Here's how the part is built. I have some questions about the finished solid (model axes, mm). A direction names the side the tool comes from. Round coordinates to 2 decimals unless told otherwise and drop trailing zeros. Order: outer loops, then holes, each group sorted by start corner. A loop starts at its lowest first (then second) coordinate and runs counter-clockwise, first axis right, second up. Notation, with made-up numbers: (35.25, 11) - (81.25, 11) arc R12 cw to (81.25, 21) - close; hole circle Ø9 at (77.25, 29.5). An arc over 180 degrees is marked (long way). Answer as a JSON object with one key per item and string values.
```python
from build123d import *
from build123d.topology import SkipClean

# Parameters (mm, degrees)
CROQUIS1_R              = 1.717841821
CROQUIS1_R_2            = 1.259750669
CROQUIS1_W              = 27.485469141
CROQUIS1_H              = 14.887962451
SALIENTE_EXTRUIR1_DEPTH = 5
SALIENTE_EXTRUIR2_START = -5
SALIENTE_EXTRUIR2_DEPTH = 5
CORTAR_EXTRUIR1_DEPTH   = 5
CORTAR_EXTRUIR2_DEPTH   = 2
CUT_EXTRUDE2_DEPTH      = 83.704538261


with BuildPart() as part:
    # Croquis1 → Saliente-Extruir1 (new body)
    with BuildSketch(Plane(origin=(0, 0, -2.5), x_dir=(-1, 0, 0), z_dir=(0, 0, -1))):
        with BuildLine():
            Line((2.183126414, 10.199004786), (2.457799007, 10.747834714))
            ThreePointArc((2.457799007, 10.747834714), (3.150356623, 11.03498533), (3.533498829, 10.390552574))
            Line((3.533498829, 10.390552574), (3.410556906, 9.704532228))
            Line((3.410556906, 9.704532228), (36.957948904, -3.17310503))
            ThreePointArc((36.957948904, -3.17310503), (40.309989238, -4.118478177), (43.778179918, -4.437160132))
            Line((43.778179918, -4.437160132), (75.884737747, -4.437160132))
            ThreePointArc((75.884737747, -4.437160132), (79.123931349, -3.095442211), (80.46564927, 0.143751392))
            Line((80.46564927, 0.143751392), (80.46564927, 13.886485962))
            ThreePointArc((80.46564927, 13.886485962), (79.123931349, 17.125679564), (75.884737747, 18.467397485))
            Line((75.884737747, 18.467397485), (43.778179918, 18.467397485))
            ThreePointArc((43.778179918, 18.467397485), (38.923372817, 17.631925595), (34.62713443, 15.221634951))
            ThreePointArc((34.62713443, 15.221634951), (27.84817952, 12.197288027), (20.46564927, 12.971336544))
            Line((20.46564927, 12.971336544), (6.293279019, 18.411599775))
            Line((6.293279019, 18.411599775), (6.008822105, 17.843219559))
            ThreePointArc((6.008822105, 17.843219559), (5.316264489, 17.556068943), (4.933122282, 18.200501699))
            Line((4.933122282, 18.200501699), (5.041383533, 18.804603367))
            ThreePointArc((5.041383533, 18.804603367), (4.263160644, 18.876341405), (3.484068945, 18.814751339))
            Line((3.484068945, 18.814751339), (3.584448287, 18.209290101))
            ThreePointArc((3.584448287, 18.209290101), (3.192940304, 17.56990522), (2.504183677, 17.866056933))
            Line((2.504183677, 17.866056933), (2.236686818, 18.418419815))
            ThreePointArc((2.236686818, 18.418419815), (1.564924714, 18.019029169), (0.970828021, 17.511263148))
            Line((0.970828021, 17.511263148), (1.407917802, 17.080436215))
            ThreePointArc((1.407917802, 17.080436215), (1.467002194, 16.333040361), (0.735712768, 16.167791142))
            Line((0.735712768, 16.167791142), (0.194632507, 16.457431391))
            ThreePointArc((0.194632507, 16.457431391), (-0.114078519, 15.739465714), (-0.296255461, 14.9794731))
            Line((-0.296255461, 14.9794731), (0.310591317, 14.887841716))
            ThreePointArc((0.310591317, 14.887841716), (0.797699855, 14.317914702), (0.303205335, 13.754384137))
            Line((0.303205335, 13.754384137), (-0.304784058, 13.670669023))
            ThreePointArc((-0.304784058, 13.670669023), (-0.132526888, 12.9083668), (0.16680132, 12.18643894))
            Line((0.16680132, 12.18643894), (0.711610253, 12.469003179))
            ThreePointArc((0.711610253, 12.469003179), (1.440684032, 12.294237755), (1.371864517, 11.547675365))
            Line((1.371864517, 11.547675365), (0.929197275, 11.122581216))
            ThreePointArc((0.929197275, 11.122581216), (1.516626257, 10.607115987), (2.183126414, 10.199004786))
        make_face()
        with Locations(Location((46.05155145, 7.015118677, 0), (0, 0, 180))):
            Circle(CROQUIS1_R, mode=Mode.SUBTRACT)
        with Locations(Location((77.659840962, 7.015118677, 0), (0, 0, 180))):
            Circle(CROQUIS1_R, mode=Mode.SUBTRACT)
        with Locations(Location((4.233310556, 14.295527136, 0), (0, 0, 180))):
            Circle(CROQUIS1_R_2, mode=Mode.SUBTRACT)
        with Locations((61.855696206, 7.015118677)):
            Rectangle(CROQUIS1_W, CROQUIS1_H, mode=Mode.SUBTRACT)
    extrude(amount=-SALIENTE_EXTRUIR1_DEPTH)

    # Croquis2 → Saliente-Extruir2 (add)
    with BuildSketch(Plane.XY.offset(2.5).offset(SALIENTE_EXTRUIR2_START)):
        with BuildLine():
            Line((-43.778179918, -4.437160132), (-75.884737747, -4.437160132))
            ThreePointArc((-75.884737747, -4.437160132), (-79.123931349, -3.095442211), (-80.46564927, 0.143751392))
            Line((-80.46564927, 0.143751392), (-80.46564927, 13.886485962))
            ThreePointArc((-80.46564927, 13.886485962), (-79.123931349, 17.125679564), (-75.884737747, 18.467397485))
            Line((-75.884737747, 18.467397485), (-43.778179918, 18.467397485))
            Line((-43.778179918, 18.467397485), (-43.778179918, -4.437160132))
        make_face()
    extrude(amount=SALIENTE_EXTRUIR2_DEPTH)

    # Croquis3 → Cortar-Extruir1 (cut)
    with BuildSketch(Plane.XY.offset(2.5)):
        with BuildLine():
            Line((-68.86564927, 10.615118677), (-63.46564927, 10.110118677))
            Line((-63.46564927, 10.110118677), (-63.46564927, 3.920118677))
            Line((-63.46564927, 3.920118677), (-68.86564927, 3.415118677))
            ThreePointArc((-68.86564927, 3.415118677), (-72.46564927, 7.015118677), (-68.86564927, 10.615118677))
        make_face()
    extrude(amount=-CORTAR_EXTRUIR1_DEPTH, mode=Mode.SUBTRACT)

    # Croquis4 → Cortar-Extruir2 (cut)
    with BuildSketch(Plane.XY.offset(2.5)):
        with BuildLine():
            Line((-54.77859891, 9.608381518), (-69.913267682, 10.700035319))
            ThreePointArc((-69.913267682, 10.700035319), (-73.947018097, 7.015118677), (-69.913267682, 3.330202034))
            Line((-69.913267682, 3.330202034), (-54.77859891, 4.421855836))
            ThreePointArc((-54.77859891, 4.421855836), (-52.36564927, 7.015118677), (-54.77859891, 9.608381518))
        make_face()
    extrude(amount=-CORTAR_EXTRUIR2_DEPTH, mode=Mode.SUBTRACT)

    # Sketch2 → Cut-Extrude2 (cut, through all)
    with SkipClean():  # the faces are left unmerged after this step: merging them gives an invalid solid
        with BuildSketch(Plane.XY.offset(0.5)):
            with BuildLine():
                Line((-69.913267682, 10.700035319), (-68.86564927, 10.615118677))
                ThreePointArc((-68.86564927, 10.615118677), (-72.46564927, 7.015118677), (-68.86564927, 3.415118677))
                Line((-68.86564927, 3.415118677), (-69.913267682, 3.330202034))
                ThreePointArc((-69.913267682, 3.330202034), (-73.947018097, 7.015118677), (-69.913267682, 10.700035319))
            make_face()
        extrude(amount=-CUT_EXTRUDE2_DEPTH, mode=Mode.SUBTRACT)


solid = part.part
```
1. For faces 4 (the face through (-38.989, 17.655, -0.035)), 5 (the face through (-66.203, 10.366, -0.979)), 6 (the face through (-62.24, 10.147, 1.514)), which set-ups out of +Z, -Z, +X, -X, +Y, -Y let a thin tool reach every point of the face, with its end or its side?
Responses:
{"face 4": "+Z, -Z, +Y", "face 5": "+Z, -Z", "face 6": "+Z"}
2. Imagine slicing it at D-D (z = -0.3). Give the number of separate pieces and of enclosed holes in the cut face, plus the area to 3 significant figures.
Responses:
{"separate pieces": "1", "enclosed holes": "2", "area": "1,310 mm2"}
3. Imagine slicing it at A-A (x = -66.5). List the corners of the cut face in (y, z) for me, plus the area to 3 significant figures.
Responses:
{"outline": "(-4.44, -2.5) - (3.64, -2.5) - (3.64, 0.5) - (3.58, 0.5) - (3.58, 2.5) - (-4.44, 2.5) - close; (10.39, -2.5) - (18.47, -2.5) - (18.47, 2.5) - (10.45, 2.5) - (10.45, 0.5) - (10.39, 0.5) - close", "area": "80.5 mm2"}
4. Imagine slicing it at C-C (x = -50). List the corners of the cut face in (y, z) for me.
Responses:
{"outline": "(-4.44, -2.5) - (18.47, -2.5) - (18.47, 2.5) - (-4.44, 2.5) - close"}
5. If I drill on L1, parallel to Y at x = -69, z = -0.7; L2, parallel to Y at x = -55, z = -0.2; L3, parallel to Y at x = -72.5, z = -0.25, over which ranges is the centre line in solid material (lowest first)? Write a range as [from, to].
Responses:
{"L1": "[-4.44, 3.4], [10.63, 18.47]", "L2": "[-4.44, 18.47]", "L3": "[-4.44, 4.08], [9.95, 18.47]"}
6. Thinking about a two-plate mould opening in X: for faces 1 (the face through (-27.952, 12.214, -0.035)), 2 (the face through (-48, 7, -2.5)), 3 (the face through (0.136, 12.919, -0.035)), which applies, pulls with the +X half, pulls with the -X half, needs draft (parallel to the pull), parting line crosses it, or undercut?
Responses:
{"face 1": "undercut", "face 2": "needs draft", "face 3": "pulls with the +X half"}
7. Imagine slicing it at B-B (y = 6.75). List the corners of the cut face in (x, z) for me, plus the area to 3 significant figures.
Responses:
{"outline": "(-80.47, -2.5) - (-73.94, -2.5) - (-73.94, 2.5) - (-80.47, 2.5) - close; (-63.47, -2.5) - (-11.11, -2.5) - (-11.11, 2.5) - (-52.38, 2.5) - (-52.38, 0.5) - (-63.47, 0.5) - close", "area": "272 mm2"}
8. For P1, Ø4.5, axis at x = -70.25, y = 7.02, coming from the +Z side; P2, Ø1, axis at x = -36, z = 0.5, coming from the -Y side; P3, Ø2.5, axis at x = -67.5, z = 0, coming from the +Y side, each with a flat end and sliding along its axis, tell me the tip position at first contact or that it passes through.
Responses:
{"P1": "through", "P2": "y = -3", "P3": "y = 18.47"}
